from build123d import *

# Parameters (mm, degrees)
F0_W     = 101.6
F0_H     = 50.8
F1_DEPTH = 25.4
F2_R     = 6.35
F3_DEPTH = 25.401
F4_W     = 19.05
F4_H     = 38.1
F6_R     = 5.08
F7_W     = 7.721651
F7_H     = 6.35


with BuildPart() as f1:
    # F0 (on Top) → F1 (new body)
    with BuildSketch(Plane.XY):
        Rectangle(F0_W, F0_H)
    extrude(amount=F1_DEPTH)

    # F2 (on face) → F3 (cut, through all)
    with BuildSketch(Plane.XY.offset(25.4)):
        with Locations((-38.1, 12.7)):
            Circle(F2_R)
        with Locations((38.1, 12.7)):
            Circle(F2_R)
        with Locations((-38.1, -12.7)):
            Circle(F2_R)
        with Locations((38.1, -12.7)):
            Circle(F2_R)
    extrude(amount=-F3_DEPTH, mode=Mode.SUBTRACT)

    # F4 (on Front) → F5 (revolve)
    with BuildSketch(Plane.XZ):
        with Locations((-9.525, 44.45)):
            Rectangle(F4_W, F4_H)
    revolve(axis=Axis((0, 0, 44.45), (0, 0, 1)))

    # F6
    f6_edges = [f1.edges().sort_by_distance(p)[0] for p in [
        (0, -25.4, 25.4),
        (0, -25.4, 0),
        (0, 25.4, 25.4),
        (0, 25.4, 0),
    ]]
    fillet(f6_edges, radius=F6_R)

    # F7 (on Front) → F8 (revolve, cut)
    with BuildSketch(Plane.XZ):
        with Locations((-19.100825, 41.275)):
            Rectangle(F7_W, F7_H)
    revolve(axis=Axis((0, 0, 63.5), (0, 0, -1)), mode=Mode.SUBTRACT)


solid = f1.part
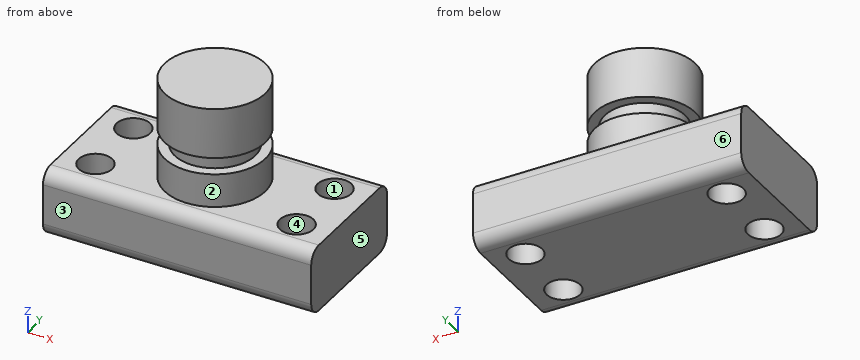
Read the model definition and answer for the solid it produces. Units are mm, in the model's axes. Face numbers are marked on the shaded views. A direction names the side the tool comes from. Give positions to 0.01 mm unless a question says otherwise; leave off trailing zeros. Loops run counter-clockwise (first coordinate to the right, second up) from the corner with the lowest first, then second, coordinate; pieces in that order, holes last. Notation, with made-up numbers: M 79.5,11.25 L 113.5,11.25 A17 cw 113.5,17.25 Z; hole C 75,-33.5 d4. An arc over 180 degrees is marked long. Write each question's results on one line, items separated by ' | '.
1. A tool of negligible diameter and unlimited length cuts with its end or side. For the marked faces 1 and 2, from which of +Z, -Z, +X, -X, +Y, -Y can it reach the whole face along a straight path? Write none if from no direction.
Values:
face 1: +Z, -Z | face 2: +Z
2. The mould has two halves that part along Y. Classify the marked faces 3, 4, 5 and 6: pulls with the +Y half, pulls with the -Y half, needs draft (parallel to the pull), parting line crosses it, or undercut.
Values:
face 3: pulls with the -Y half | face 4: undercut | face 5: needs draft | face 6: pulls with the +Y half
3. Straight lines are drawn through the part: line 1 (Y direction, x = 38.1, z = 13.75); line 2 (X direction, y = 11, z = 11.5); line 3 (Y direction, x = 36, z = 5). For each, find the intervals that lie inside material, in ascending order. Write a range as [from, to].
Values:
line 1: y = [-25.4, -19.05], [-6.35, 6.35], [19.05, 25.4] | line 2: x = [-50.8, -44.22], [-31.98, 31.98], [44.22, 50.8] | line 3: y = [-25.4, -18.69], [-6.71, 6.71], [18.69, 25.4]
4. Section A-A on x = -38.1 is taken. Give the vertices of the cut face in (y, z).
Values:
outline: M -25.4,5.08 A5.08 ccw -20.32,0 L -19.05,0 L -19.05,25.4 L -20.32,25.4 A5.08 ccw -25.4,20.32 Z; M -6.35,0 L 6.35,0 L 6.35,25.4 L -6.35,25.4 Z; M 19.05,0 L 20.32,0 A5.08 ccw 25.4,5.08 L 25.4,20.32 A5.08 ccw 20.32,25.4 L 19.05,25.4 Z
5. Section B-B on y = 12.7 is taken. Give the vertices of the cut face in (x, z).
Values:
outline: M -50.8,0 L -44.45,0 L -44.45,25.4 L -50.8,25.4 Z; M -31.75,0 L 31.75,0 L 31.75,25.4 L 14.2,25.4 L 14.2,38.1 L 8.42,38.1 L 8.42,44.45 L 14.2,44.45 L 14.2,63.5 L -14.2,63.5 L -14.2,44.45 L -8.42,44.45 L -8.42,38.1 L -14.2,38.1 L -14.2,25.4 L -31.75,25.4 Z; M 44.45,0 L 50.8,0 L 50.8,25.4 L 44.45,25.4 Z
6. Section D-D on y = 0 is taken. Give the vertices of the cut face in (x, z).
Values:
outline: M -50.8,0 L 50.8,0 L 50.8,25.4 L 19.05,25.4 L 19.05,38.1 L 15.24,38.1 L 15.24,44.45 L 19.05,44.45 L 19.05,63.5 L -19.05,63.5 L -19.05,44.45 L -15.24,44.45 L -15.24,38.1 L -19.05,38.1 L -19.05,25.4 L -50.8,25.4 Z
7. Given pin 1 (6 mm diameter, centred on y = 2.5, z = 38, fed in from -X); pin 2 (7.5 mm diameter, centred on x = 38.1, y = -12.7, fed in from -Z); pin 3 (20.5 mm diameter, centred on x = -38.1, y = -12.7, fed in from +Z); pin 4 (6 mm diameter, centred on x = 25.5, y = 16, fed in from -Z), each flat-ended and moving along its own axis, determine where each tip first touches the part or whether it passes through.
Values:
pin 1: stops at x = -19.05 | pin 2: passes through | pin 3: stops at z = 25.4 | pin 4: stops at z = 0
8. Section C-C on x = 27 is taken. Give the vertices of the cut face in (y, z).
Values:
outline: M -25.4,5.08 A5.08 ccw -20.32,0 L 20.32,0 A5.08 ccw 25.4,5.08 L 25.4,20.32 A5.08 ccw 20.32,25.4 L -20.32,25.4 A5.08 ccw -25.4,20.32 Z
